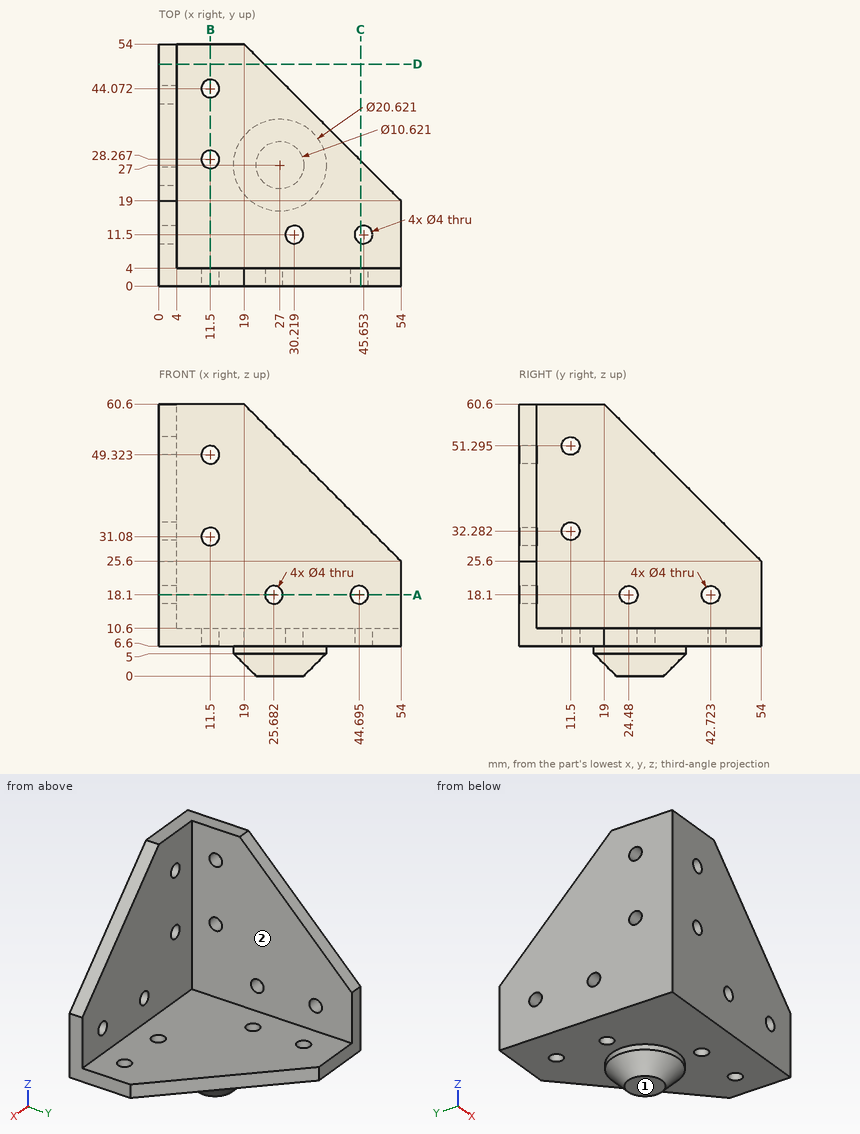
Verification items for this drawing (mm, ordinates from the low corner). A direction names the side the tool comes from. Coordinates: 2 decimals unless noted, no trailing zeros. Loops run counter-clockwise (first coordinate to the right, second up) from the corner with the lowest first, then second, coordinate; pieces in that order, holes last.
Item 1: Sectioned sample at C-C, the plane x = 45. Record the boundary of the cut face in (y, z), then the cut area to 3 significant figures.
Item 2: Thickness scan on line 1 (Z direction, x = 1.25, y = 11.5) (1 decimal); line 2 (Y direction, x = 2, z = 18) (1 decimal); line 3 (Z direction, x = 11, y = 3) (1 decimal). Record the ranges inside material, lowest first.
Item 3: Sectioned sample at A-A, the plane z = 18.1. Record the boundary of the cut face in (x, y) (1 decimal).
Item 4: Access from +Z, -Z, +X, -X, +Y, -Y to the whole of each face (thin tool, end or side, straight path). Record for the marked faces 1 and 2.
Item 5: Go/stop test with flat-tipped pins: pin 1 Ø6.5 at (y, z) = (42.72, 18.1) entering from +X; pin 2 Ø25 at (x, z) = (21.5, 30.5) entering from +Y; pin 3 Ø5 at (x, y) = (30.22, 11.5) entering from +Z. Record where each tip stops, or that it passes through.
Item 6: Sectioned sample at D-D, the plane y = 49.5. Record the boundary of the cut face in (x, z).
Item 7: Sectioned sample at B-B, the plane x = 11.5. Record the boundary of the cut face in (y, z), then the cut area to 3 significant figures.
Check result:
1. outline: (0, 6.6) - (9.61, 6.6) - (9.61, 10.6) - (4, 10.6) - (4, 16.12) - (0, 16.12) - close; (0, 20.08) - (4, 20.08) - (4, 34.6) - (0, 34.6) - close; (13.39, 6.6) - (28, 6.6) - (28, 10.6) - (13.39, 10.6) - close
1. area: 177 mm2
2. line 1: z = 6.6 to 30.3, 34.3 to 49.3, 53.3 to 60.6
2. line 2: y = 0 to 22.5, 26.5 to 40.7, 44.7 to 54
2. line 3: z = 6.6 to 29.1, 33 to 47.4, 51.3 to 60.6
3. outline: (0, 0) - (23.7, 0) - (23.7, 4) - (4, 4) - (4, 22.5) - (0, 22.5) - close; (0, 26.5) - (4, 26.5) - (4, 40.7) - (0, 40.7) - close; (0, 44.7) - (4, 44.7) - (4, 54) - (0, 54) - close; (27.7, 0) - (42.7, 0) - (42.7, 4) - (27.7, 4) - close; (46.7, 0) - (54, 0) - (54, 4) - (46.7, 4) - close
4. face 1: -Z, +X, -X, +Y, -Y
4. face 2: +Z, +X, +Y
5. pin 1: stops at x = 4
5. pin 2: stops at y = 4
5. pin 3: stops at z = 10.6
6. outline: (0, 6.6) - (23.5, 6.6) - (23.5, 10.6) - (4, 10.6) - (4, 30.1) - (0, 30.1) - close
7. outline: (0, 6.6) - (26.27, 6.6) - (26.27, 10.6) - (4, 10.6) - (4, 29.08) - (0, 29.08) - close; (0, 33.08) - (4, 33.08) - (4, 47.32) - (0, 47.32) - close; (0, 51.32) - (4, 51.32) - (4, 60.6) - (0, 60.6) - close; (30.27, 6.6) - (42.07, 6.6) - (42.07, 10.6) - (30.27, 10.6) - close; (46.07, 6.6) - (54, 6.6) - (54, 10.6) - (46.07, 10.6) - close
7. area: 352 mm2
